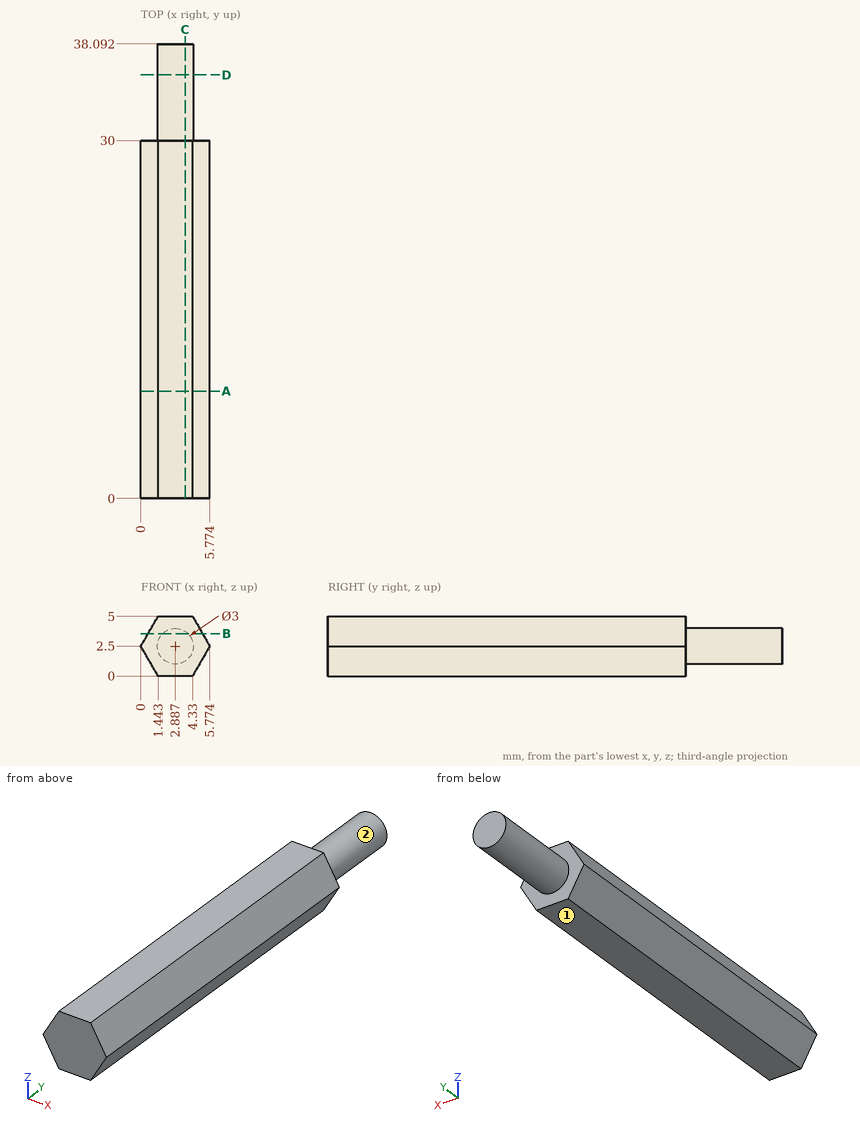
Check sheet for the drawn part. Datum: minimum x, y, z corner. Units: mm. A direction names the side the tool comes from. Give positions to 0.01 mm unless a question says otherwise; leave off trailing zeros. Write each loop counter-clockwise with the first axis right and the second up, starting at its lowest first coordinate (ties: lowest second). Pieces come first, ordered by that corner, then holes.
(1) Material ranges on line 1 (Y direction, x = 0.4, z = 2.35); line 2 (Z direction, x = 5, y = 11.5); line 3 (X direction, y = 35, z = 3.55) (1 decimal), recorded low to high.
(2) Access from +Z, -Z, +X, -X, +Y, -Y to the whole of each face (thin tool, end or side, straight path). Record for the marked faces 1 and 2.
(3) Cross-section at C-C (x = 3.7). Enter the section's corners in (y, z), plus the area to 3 significant figures.
(4) Cross-section at B-B (z = 3.55). Enter the section's corners in (x, y) (1 decimal).
(5) Cross-section at A-A (y = 9). Enter the section's corners in (x, z).
(6) Cross-section at D-D (y = 35.5). Enter the section's corners in (x, z).
Worked out:
1. line 1: y = 0 to 30
1. line 2: z = 1.16 to 3.84
1. line 3: x = 1.8 to 4
2. face 1: -Z, +X, -X, +Y, -Y
2. face 2: +Y
3. outline: (0, 0) - (30, 0) - (30, 1.24) - (38.09, 1.24) - (38.09, 3.76) - (30, 3.76) - (30, 5) - (0, 5) - close
3. area: 170 mm2
4. outline: (0.6, 0) - (5.2, 0) - (5.2, 30) - (4, 30) - (4, 38.1) - (1.8, 38.1) - (1.8, 30) - (0.6, 30) - close
5. outline: (0, 2.5) - (1.44, 0) - (4.33, 0) - (5.77, 2.5) - (4.33, 5) - (1.44, 5) - close
6. outline: circle Ø3 at (2.89, 2.5)
